Work out the finished part from the listing and answer in its coordinate system (mm). A direction names the side the tool comes from. Round coordinates to 2 decimals unless told otherwise and drop trailing zeros. Loops run counter-clockwise (first coordinate to the right, second up) from the corner with the lowest first, then second, coordinate; pieces in that order, holes last.
```python
from build123d import *

# Parameters (mm, degrees)
CHANFRO4_SIZE   = 0.55
CHANFRO4_SIZE_2 = 1.79896894


with BuildPart() as part:
    # Esboço1 → Revolução1 (revolve)
    with BuildSketch(Plane.XY, mode=Mode.PRIVATE) as revolu_o1_sk:
        Polygon((4.16, 1), (4.16, 4.45), (16.84, 4.45), (16.84, 4.69), (3.2, 4.69), (3.2, 4.15), (1.2, 4.15), (1.2, 4.69), (0, 4.69), (0, 2.25), (3, 2.25), (3, 1), align=None)
    revolve(revolu_o1_sk.sketch.rotate(Axis((0, 0, 0), (1, 0, 0)), 90), axis=Axis((0, 0, 0), (1, 0, 0)))

    # Chanfro4
    # the kernel refuses this chamfer: 1.79896894, 0.55 mm, written as the material it adds along each edge
    with BuildSketch(Plane(origin=(3.2, 0, 0), x_dir=(0, 0, 1), z_dir=(0, 1, 0))) as chanfro4_piece_1_section:
        Polygon((4.15 + CHANFRO4_SIZE, 0), (4.15, -CHANFRO4_SIZE_2), (4.15, 0), align=None)
    chanfro4_piece_1 = revolve(axis=Axis((3.2, 0, 0), (1, 0, 0)), mode=Mode.PRIVATE)
    chanfro4_piece_1 = chanfro4_piece_1 & Plane(origin=(2.25712916, 0, 0), x_dir=(0, 0, 1), z_dir=(-1, 0, 0)) * Cylinder(4.69, 19, mode=Mode.PRIVATE)
    add(chanfro4_piece_1)


solid = part.part
```
1. Find section A-A (z = 0). Write down the section's boundary in (x, y).
Answer key:
outline: (0, -4.69) - (1.2, -4.69) - (1.2, -4.15) - (1.4, -4.15) - (3.17, -4.69) - (16.84, -4.69) - (16.84, -4.45) - (4.16, -4.45) - (4.16, -1) - (3, -1) - (3, -2.25) - (0, -2.25) - close; (0, 2.25) - (3, 2.25) - (3, 1) - (4.16, 1) - (4.16, 4.45) - (16.84, 4.45) - (16.84, 4.69) - (3.17, 4.69) - (1.4, 4.15) - (1.2, 4.15) - (1.2, 4.69) - (0, 4.69) - close
2. Which of the six approach directions +Z, -Z, +X, -X, +Y, -Y give full straight-line access (tool end or side, diameter ignored) to faces 1 (the face through (3, 1, -1)), 2 (the face through (9.91, 4.65, -0.61)), 3 (the face through (10.59, -3.01, -3.28))?
Answer key:
face 1: -X
face 2: +X, -X
face 3: +X
3. Given pin 1 (2 mm diameter, centred on y = -3, z = 1, fed in from +X), flat-ended and moving along its own axis, determine where the tip first touches the part or whether it passes through.
Answer key:
pin 1: stops at x = 4.16
4. Find section C-C (x = 9.75). Write down the section's boundary in (y, z), then the cut area to 3 significant figures.
Answer key:
outline: circle Ø9.38 at (0, 0); hole circle Ø8.9 at (0, 0)
area: 6.89 mm2
5. Consider probe 1 along Y at (x, z) = (10.5, 0); probe 2 along X at (y, z) = (-1.25, 3.5); probe 3 along Y at (x, z) = (1.5, -1.75). Determine where each line is inside the solid, lowest interval first.
Answer key:
probe 1: y = -4.69 to -4.45, 4.45 to 4.69
probe 2: x = 0 to 4.16
probe 3: y = -3.8 to -1.41, 1.41 to 3.8
6. Determine the mould class of faces 4 (the face through (1.2, 4, -2)), 5 (the face through (4.16, 1, -1)), 6 (the face through (0.592, -1.409, 4.473)) for opening direction X: +X half, -X half, draft (parallel to the pull), parting line (faces both ways), or undercut.
Answer key:
face 4: undercut
face 5: +X half
face 6: draft
